```python
from build123d import *

# Parameters (mm, degrees)
F0_R          = 5.3213500883
F1_DEPTH      = 12.7
F3_DEPTH      = 38.1
F3_DEPTH_BACK = 38.1
F5_DEPTH      = 20.9411715547
F5_DEPTH_BACK = 20.9411715547


with BuildPart() as f1:
    # F0 (on Top) → F1 (new body)
    with BuildSketch(Plane.XY):
        with BuildLine():
            Line((62.1395111084, 20.9401715547), (0, 20.9401715547))
            Line((0, 20.9401715547), (-62.1395111084, 20.9401715547))
            ThreePointArc((-62.1395111084, 20.9401715547), (-76.9464484139, 14.8069373055), (-83.0796826631, 0))
            ThreePointArc((-83.0796826631, 0), (-76.9464484139, -14.8069373055), (-62.1395111084, -20.9401715547))
            Line((-62.1395111084, -20.9401715547), (0, -20.9401715547))
            Line((0, -20.9401715547), (62.1395111084, -20.9401715547))
            ThreePointArc((62.1395111084, -20.9401715547), (76.9464484139, -14.8069373055), (83.0796826631, 0))
            ThreePointArc((83.0796826631, 0), (76.9464484139, 14.8069373055), (62.1395111084, 20.9401715547))
        make_face()
        with Locations((-62.1395111084, 0)):
            Circle(F0_R, mode=Mode.SUBTRACT)
        with Locations((62.1395111084, 0)):
            Circle(F0_R, mode=Mode.SUBTRACT)
    extrude(amount=F1_DEPTH)

    # F2 (on Right) → F3 (join, two sides)
    with BuildSketch(Plane.YZ) as f3_sk:
        with BuildLine():
            Line((-9.0088532658, 12.7), (0, 12.7))
            Line((0, 12.7), (9.0088532658, 12.7))
            Line((9.0088532658, 12.7), (9.0088532658, 32.3224291205))
            ThreePointArc((9.0088532658, 32.3224291205), (6.370221235, 38.6926503555), (0, 41.3312823864))
            ThreePointArc((0, 41.3312823864), (-6.370221235, 38.6926503555), (-9.0088532658, 32.3224291205))
            Line((-9.0088532658, 32.3224291205), (-9.0088532658, 12.7))
        make_face()
        with BuildLine():
            ThreePointArc((0, 29.7824291205), (-2.54, 32.3224291205), (0, 34.8624291205))
            ThreePointArc((0, 34.8624291205), (2.54, 32.3224291205), (0, 29.7824291205))
        make_face(mode=Mode.SUBTRACT)
    extrude(amount=F3_DEPTH)
    extrude(f3_sk.sketch, amount=-F3_DEPTH_BACK)

    # F4 (on Front) → F5 (cut, two sides)
    with BuildSketch(Plane.XZ) as f5_sk:
        with BuildLine():
            Line((13.5943368077, 41.3312823864), (-13.5943368077, 41.3312823864))
            Line((-13.5943368077, 41.3312823864), (-13.5943368077, 29.7987964004))
            ThreePointArc((-13.5943368077, 29.7987964004), (-9.6126477425, 20.1861486579), (0, 16.2044595927))
            ThreePointArc((0, 16.2044595927), (9.6126477425, 20.1861486579), (13.5943368077, 29.7987964004))
            Line((13.5943368077, 29.7987964004), (13.5943368077, 41.3312823864))
        make_face()
    extrude(amount=-F5_DEPTH, mode=Mode.SUBTRACT)
    extrude(f5_sk.sketch, amount=F5_DEPTH_BACK, mode=Mode.SUBTRACT)


solid = f1.part
```
For this review, take the finished solid that the model builds, in its own axes (mm). A direction names the side the tool comes from. Coordinates: 2 decimals unless noted, no trailing zeros. Loops run counter-clockwise (first coordinate to the right, second up) from the corner with the lowest first, then second, coordinate; pieces in that order, holes last.
1. For line 1 (X direction, y = -2, z = 30); line 2 (Z direction, x = 31.5, y = 0); line 3 (Z direction, x = -56.5, y = 14.5), list the stretches that pass through material, from the lowest coordinate up.
2. Mouldability with a two-part tool opening along Y and no side actions: class faces 1 (the cylindrical face through (-67.456, 0.234, 6.261)), 2 (the flat face through (-38.1, 0, 27)), 3 (the flat face through (1, 20.94, 6)) as +Y half, -Y half, draft (parallel to the pull), parting line (faces both ways), or undercut.
3. For faces 4 (the flat face through (13.594, 0.1, 35.5)), 5 (the flat face through (-1, 0, 0)), 6 (the flat face through (1, -9.009, 16)), 7 (the flat face through (38.1, 0, 27)), 8 (the flat face through (-1, 9.009, 16)), list the 3-axis set-ups (+Z, -Z, +X, -X, +Y, -Y) from which the entire face can be reached by the end or side of a thin tool; tool diameter is ignored.
4. Add section C-C, the plane z = 18. Give the boundary of the cut face in (x, y).
5. Insertion check: P1, Ø6, axis at x = -15, z = 18.5, coming from the -Y side; P2, Ø3, axis at y = -7.5, z = 14, coming from the -X side; P3, Ø21.5, axis at x = 14.5, z = 24, coming from the +Y side; P4, Ø1, axis at x = 64, y = -4, coming from the -Z side. Each pin has a flat end and moves straight along its axis. Give the tip position at first contact, or say it passes through.
6. Add section A-A, the plane z = 5. Give the boundary of the cut face in (x, y), then the cut area to 3 significant figures.
7. Add section B-B, the plane x = 22.5. Give the boundary of the cut face in (y, z), then the cut area to 3 significant figures.
8. Add section D-D, the plane x = 0. Give the boundary of the cut face in (y, z), then the cut area to 3 significant figures.
Result:
1. line 1: x = -38.1 to -13.59, 13.59 to 38.1
1. line 2: z = 0 to 29.78, 34.86 to 41.33
1. line 3: z = 0 to 12.7
2. face 1: undercut
2. face 2: draft
2. face 3: +Y half
3. face 4: +Z, +Y, -Y
3. face 5: -Z, +X, -X, +Y, -Y
3. face 6: +Z, +X, -X, -Y
3. face 7: +Z, +X, +Y, -Y
3. face 8: +Z, +X, -X, +Y
4. outline: (-38.1, -9.01) - (-6.75, -9.01) - (-6.75, 9.01) - (-38.1, 9.01) - close; (6.75, -9.01) - (38.1, -9.01) - (38.1, 9.01) - (6.75, 9.01) - close
5. P1: stops at y = -9.01
5. P2: stops at x = -81.96
5. P3: stops at y = 9.01
5. P4: passes through
6. outline: (-62.14, -20.94) - (62.14, -20.94) arc R20.94 ccw to (62.14, 20.94) - (-62.14, 20.94) arc R20.94 ccw to start; hole circle Ø10.64 at (-62.14, 0); hole circle Ø10.64 at (62.14, 0)
6. area: 6,400 mm2
7. outline: (-20.94, 0) - (20.94, 0) - (20.94, 12.7) - (9.01, 12.7) - (9.01, 32.32) arc R9.01 ccw to (-9.01, 32.32) - (-9.01, 12.7) - (-20.94, 12.7) - close; hole circle Ø5.08 at (0, 32.32)
7. area: 993 mm2
8. outline: (-20.94, 0) - (20.94, 0) - (20.94, 12.7) - (9.01, 12.7) - (9.01, 16.2) - (-9.01, 16.2) - (-9.01, 12.7) - (-20.94, 12.7) - close
8. area: 595 mm2
